Solid Edge part; units mm, degrees
sketch "Sketch1" plane through (0, 0, 0) normal (0, -1, 0) x (1, 0, 0)
  arc A0 (14.2007, 32.9926) -> (15.3207, 34.1126) centre (14.2007, 34.1126) ccw
  line L0 (15.3207, 34.1126) -> (15.3207, 36.3526)
  arc A1 (15.3207, 36.3526) -> (14.2007, 37.4726) centre (14.2007, 36.3526) ccw
  line L1 (14.2007, 37.4726) -> (13.6407, 37.4726)
  arc A2 (13.6407, 37.4726) -> (12.4707, 36.3026) centre (13.6407, 36.3026) ccw
  line L2 (12.4707, 36.3026) -> (12.4707, 34.1626)
  arc A3 (13.6407, 32.9926) -> (12.4707, 34.1626) centre (13.6407, 34.1626) cw
  line L3 (13.6407, 32.9926) -> (14.2007, 32.9926)
revolve "RevolvedProtrusion1" add sketch "Sketch1" angle 360 about axis through (13.9207, 0, -4.0074) along (1, 0, 0)
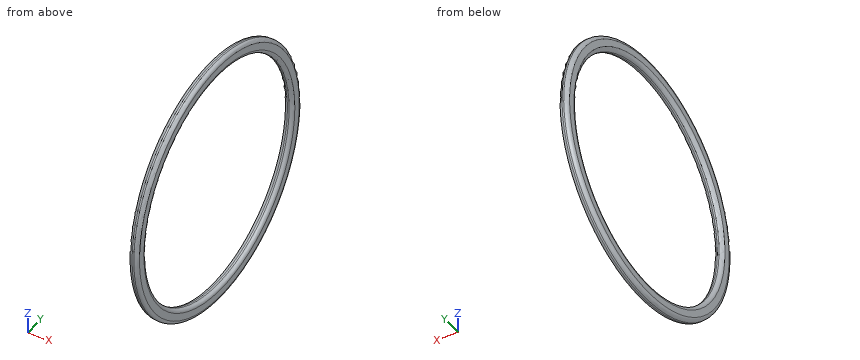
Can you work these out from the model? Positions are in its coordinate system, mm. Coordinates: 2 decimals unless noted, no trailing zeros. Loops run counter-clockwise (first coordinate to the right, second up) from the corner with the lowest first, then second, coordinate; pieces in that order, holes last.
1) Imagine slicing it at A-A on y = 0. List the corners of the cut face in (x, z) for me.
2) I need wall thicknesses on probe 1 along Z at (x, y) = (14.05, 0); probe 2 along Y at (x, z) = (14.2, -18); probe 3 along Z at (x, y) = (14.2, -18). Which ranges of each line are inside material? Lowest first, please.
3) Imagine slicing it at B-B on x = 12.9. List the corners of the cut face in (y, z) for me.
4) For pin 1 (1.5 mm diameter, centred on x = 14, z = -5, fed in from -Y); pin 2 (5 mm diameter, centred on y = 29, z = 20, fed in from +X), each with a flat end and sliding along its axis, tell me the tip position at first contact or that it passes through.
Completed:
1. outline: (12.47, -44.32) arc R1.17 ccw to (13.64, -45.49) - (14.2, -45.49) arc R1.12 ccw to (15.32, -44.37) - (15.32, -42.13) arc R1.12 ccw to (14.2, -41.01) - (13.64, -41.01) arc R1.17 ccw to (12.47, -42.18) - close; (12.47, 34.16) arc R1.17 ccw to (13.64, 32.99) - (14.2, 32.99) arc R1.12 ccw to (15.32, 34.11) - (15.32, 36.35) arc R1.12 ccw to (14.2, 37.47) - (13.64, 37.47) arc R1.17 ccw to (12.47, 36.3) - close
2. probe 1: z = -45.49 to -41.01, 32.99 to 37.47
2. probe 2: y = -39.05 to -34.25, 34.25 to 39.05
2. probe 3: z = -41.38 to -36.33, 28.32 to 33.36
3. outline: circle Ø82.43 at (0, -4.01); hole circle Ø74.53 at (0, -4.01)
4. pin 1: stops at y = -41.48
4. pin 2: stops at x = 15.32
